Part model, mm, in its own coordinate system. Face numbers are marked on the shaded views. A direction names the side the tool comes from. Coordinates: 2 decimals unless noted, no trailing zeros. Order: outer loops, then holes, each group sorted by start corner. A loop starts at its lowest first (then second) coordinate and runs counter-clockwise, first axis right, second up.
```python
from build123d import *

# Parameters (mm, degrees)
F2_R     = 1
F3_SIZE  = 1.5
F5_DEPTH = 7


with BuildPart() as f1:
    # F0 (on Top) → F1 (revolve)
    with BuildSketch(Plane.XY):
        Polygon((-30.745121, 12), (-30.745121, 0), (45.254879, 0), (45.254879, 8), (-14.745121, 8), (-14.745121, 12), align=None)
    revolve(axis=Axis((0.541581, 0, 0), (1, 0, 0)))

    # F2
    f2_edges = [f1.edges().sort_by_distance(p)[0] for p in [
        (-30.745121, -12, 0),
    ]]
    fillet(f2_edges, radius=F2_R)

    # F3
    f3_edges = [f1.edges().sort_by_distance(p)[0] for p in [
        (45.254879, -8, 0),
    ]]
    chamfer(f3_edges, length=F3_SIZE)

    # F4 (on face) → F5 (cut)
    with BuildSketch(Plane(origin=(-30.745121, 0, 0), x_dir=(0, -1, 0), z_dir=(-1, 0, 0))):
        Polygon((7, -4.041452), (7, 2.453793), (7, 4.041452), (0, 8.082904), (-7, 4.041452), (-7, 2.453793), (-7, -4.041452), (0, -8.082904), align=None)
    extrude(amount=-F5_DEPTH, mode=Mode.SUBTRACT)

    # F6 (on Front) → F7 (revolve, cut)
    with BuildSketch(Plane.XZ):
        Polygon((-29.745121, 7.082904), (-30.745121, 8.082904), (-30.745121, 0), (-29.745121, 0), align=None)
    revolve(axis=Axis((0.541581, 0, 0), (1, 0, 0)), mode=Mode.SUBTRACT)


with BuildPart() as f8_1:
    # F8: copy of F1
    add(f1.part)


solid = f1.part
```
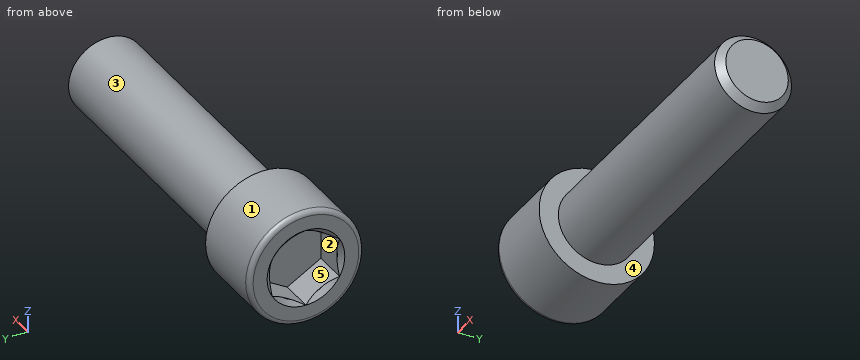
(1) Drop flat-ended pins along their axis: pin 1 (3.5 mm diameter, centred on x = -28, z = -2, fed in from -Y); pin 2 (4 mm diameter, centred on y = 1, z = 3.5, fed in from -X); pin 3 (10 mm diameter, centred on x = 31, z = -1, fed in from +Y); pin 4 (6 mm diameter, centred on x = -21.5, y = 2, fed in from -Z). Give the stop position or say it passes through.
(2) Slice it at B-B, the plane x = -16. Give the cut face in (y, z).
(3) Pull direction Z, two halves, no side cores. Call the marked faces 3, 4 and 5: +Z half, -Z half, draft (parallel to the pull), parting line (faces both ways), or undercut.
(4) Probe line 1 (X direction, y = 9.25, z = -5); line 2 (X direction, y = 3.5, z = 3.25); line 3 (Z direction, x = 22.5, y = 3.75). List the from-to ranges inside material, lowest first.
(5) Slice it at A-A, the plane z = 0. Give the cut face in (x, y).
(6) Tool access for the marked faces 1 and 2: list every direction of +Z, -Z, +X, -X, +Y, -Y with a clear straight run to the whole face (end or side of a thin tool).
Here are the results:
1. pin 1: stops at y = -12
1. pin 2: stops at x = -23.75
1. pin 3: stops at y = 8
1. pin 4: stops at z = -12
2. outline: circle Ø24 at (0, 0)
3. face 3: parting line
3. face 4: draft
3. face 5: undercut
4. line 1: x = -30.75 to -14.75
4. line 2: x = -23.75 to 45.25
4. line 3: z = -7.07 to 7.07
5. outline: (-30.75, -11) arc R1 ccw to (-29.75, -12) - (-14.75, -12) - (-14.75, -8) - (43.75, -8) - (45.25, -6.5) - (45.25, 6.5) - (43.75, 8) - (-14.75, 8) - (-14.75, 12) - (-29.75, 12) arc R1 ccw to (-30.75, 11) - (-30.75, 8.08) - (-29.75, 7.08) - (-29.75, 7) - (-23.75, 7) - (-23.75, -7) - (-29.75, -7) - (-29.75, -7.08) - (-30.75, -8.08) - close
6. face 1: +X, -X
6. face 2: -X
